Input: part model. Units: mm. Frame: model coordinates. Face numbers are marked on the shaded views. A direction names the side the tool comes from. Give positions to 0.01 mm unless a question says otherwise; leave off trailing zeros. Loops run counter-clockwise (first coordinate to the right, second up) from the corner with the lowest first, then second, coordinate; pieces in that order, holes last. Notation, with made-up numbers: M 40,55 L 46,55 A26 ccw 46,73 Z; hole C 89.5,59.25 d7. An arc over 180 degrees is marked long. Use CSV: the item, a comma, the result in double quotes. Start each with the question number.
Q1. Section A-A, the plane y = 0. Output: boundary loops of the cut face in (x, z) (3 decimals), plus the area to 3 significant figures.
Q2. Section B-B, the plane x = 13.5. Output: boundary loops of the cut face in (y, z) (3 decimals), plus the area to 3 significant figures.
Q3. Pull-direction query (Y, two-part tool) for the marked faces 1, 2 and 3; classes: released by +Y, released by -Y, zero draft, split by the parting line, or undercut.
Q4. Reachability of the marked faces 4 and 5 from +Z, -Z, +X, -X, +Y, -Y: full face, straight path, thin tool, end or side. Return the list, or none.
Q5. Material intervals for line 1 along X through (y, z) = (-10, -5); line 2 along X through (y, z) = (-26, 4.5); line 3 along Y through (x, z) = (-12.5, 6.5), sorted ascending.
Q6. Pin query (flat end, axial travel): pin 1 (8.5 mm diameter, centred on x = -25.5, y = -5, fed in from +Z); pin 2 (3 mm diameter, centred on x = 12, y = 1, fed in from +Z); pin 3 (3 mm diameter, centred on x = 15.5, y = 11, fed in from +Z). Return the tip coordinate at first contact, or that it passes through.
Q7. Section C-C, the plane x = -11. Output: boundary loops of the cut face in (y, z) (3 decimals).
from build123d import *

# Parameters (mm, degrees)
F3_DEPTH = 29.0322
F5_D     = 2.9464


with BuildPart() as f1:
    # F0 (on Front) → F1 (revolve)
    with BuildSketch(Plane.XZ):
        with BuildLine():
            Line((-33.2725646531, 12.9185590085), (-33.2725646531, -5.6210034922))
            Line((-33.2725646531, -5.6210034922), (17.0194353469, -5.6210034922))
            ThreePointArc((17.0194353469, -5.6210034922), (18.0970660814, -6.0673727577), (18.5434353469, -7.1450034922))
            Line((18.5434353469, -7.1450034922), (18.5434353469, -13.7490034922))
            ThreePointArc((18.5434353469, -13.7490034922), (18.8410148572, -14.4674239819), (19.5594353469, -14.7650034922))
            Line((19.5594353469, -14.7650034922), (28.7034353469, -14.7650034922))
            Line((28.7034353469, -14.7650034922), (28.7034353469, -12.8663534922))
            Line((28.7034353469, -12.8663534922), (23.2424353469, -12.8663534922))
            Line((23.2424353469, -12.8663534922), (23.2424353469, -2.4460034922))
            Line((23.2424353469, -2.4460034922), (-30.2245646531, -2.4460034922))
            Line((-30.2245646531, -2.4460034922), (-30.2245646531, 12.9185590085))
            Line((-30.2245646531, 12.9185590085), (-33.2725646531, 12.9185590085))
        make_face()
    revolve(axis=Axis((-6.179202348, 0, 14.4449965078), (1, 0, 0)))

    # F2 (on Front) → F3 (cut, symmetric)
    with BuildSketch(Plane.XZ):
        with BuildLine():
            Line((8.8914353469, 39.0829965078), (8.8914353469, 42.0824922621))
            Line((8.8914353469, 42.0824922621), (-33.2725646531, 42.0824922621))
            Line((-33.2725646531, 42.0824922621), (-33.2725646531, 34.5109965078))
            Line((-33.2725646531, 34.5109965078), (-33.2725646531, 7.3329965078))
            Line((-33.2725646531, 7.3329965078), (-22.8585646531, 7.3329965078))
            ThreePointArc((-22.8585646531, 7.3329965078), (-0.4079243504, 16.6323562051), (8.8914353469, 39.0829965078))
        make_face()
    extrude(amount=F3_DEPTH, both=True, mode=Mode.SUBTRACT)

    # F5 (through all)
    with Locations(Plane(origin=(18.5434353469, 0, 0), x_dir=(0, -1, 0), z_dir=(-1, 0, 0))):
        with Locations((12.573, 36.2127965078), (21.7678, 27.0179965078), (-12.573, 36.2127965078), (-21.7678, 27.0179965078), (21.7678, 1.8719965078), (12.573, -7.3228034922), (-12.573, -7.3228034922), (-21.7678, 1.8719965078)):
            Hole(F5_D / 2)


solid = f1.part
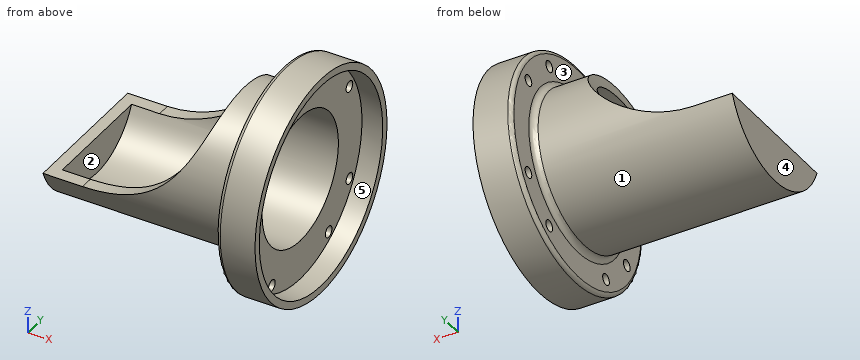
A:
1,outline,"M -33.273,-5.621 L 17.019,-5.621 A1.524 cw 18.543,-7.145 L 18.543,-13.749 A1.016 ccw 19.559,-14.765 L 28.703,-14.765 L 28.703,-12.866 L 23.242,-12.866 L 23.242,-2.446 L -30.225,-2.446 L -30.225,7.333 L -33.273,7.333 Z; M 7.932,31.336 L 23.242,31.336 L 23.242,41.756 L 28.703,41.756 L 28.703,43.655 L 19.559,43.655 A1.016 ccw 18.543,42.639 L 18.543,36.035 A1.524 cw 17.019,34.511 L 8.561,34.511 A31.75 cw Z"
1,area,"364 mm^2"
2,outline,"C 0,14.445 d40.132; hole C 0,14.445 d33.782"
2,area,"369 mm^2"
3,face 1,"split by the parting line"
3,face 2,"undercut"
3,face 3,"zero draft"
4,face 4,"+Z, -Z, -X, +Y, -Y"
4,face 5,"+X"
5,line 1,"18.54 to 23.24"
5,line 2,"18.54 to 28.7"
5,line 3,"-18.43 to -14.91, 14.91 to 18.43"
6,pin 1,"z = 0.31"
6,pin 2,"z = 34.51"
6,pin 3,"z = 32.12"
7,outline,"M -19.48,9.631 A20.066 ccw 19.48,9.631 L 16.19,9.631 A16.891 cw -16.19,9.631 Z"
